Source: CAD feature listing. Evaluate the final solid. Frame: model axes, mm. A direction names the side the tool comes from. Give positions to 0.01 mm unless a question says otherwise; leave off trailing zeros. Write each loop counter-clockwise with the first axis right and the second up, starting at its lowest first coordinate (ties: lowest second). Pieces come first, ordered by that corner, then holes. Notation, with made-up numbers: M 5.25,-1 L 46.25,-1 A11 cw 46.25,5 Z; hole C 42,-11.5 d5. An arc over 180 degrees is marked long. Use CSV: the item, a comma, the result in double quotes. Start each with the question number.
from build123d import *

# Parameters (mm, degrees)
SKETCH1_R           = 19.75
BOSS_EXTRUDE1_DEPTH = 0.55


with BuildPart() as part:
    # Sketch1 → Boss-Extrude1 (new body)
    with BuildSketch(Plane(origin=(0, 0, 0), x_dir=(0, 0, -1), z_dir=(1, 0, 0))):
        Circle(SKETCH1_R)
        with BuildLine():
            Line((5.922649731, 1), (3.872983346, 1))
            ThreePointArc((3.872983346, 1), (0, 4), (-3.872983346, 1))
            Line((-3.872983346, 1), (-5.922649731, 1))
            Line((-5.922649731, 1), (-7.077350269, 1))
            Line((-7.077350269, 1), (-7.654700538, 0))
            Line((-7.654700538, 0), (-7.077350269, -1))
            Line((-7.077350269, -1), (-5.922649731, -1))
            Line((-5.922649731, -1), (-3.872983346, -1))
            ThreePointArc((-3.872983346, -1), (0, -4), (3.872983346, -1))
            Line((3.872983346, -1), (5.922649731, -1))
            Line((5.922649731, -1), (6.5, -1))
            Line((6.5, -1), (7.077350269, -1))
            Line((7.077350269, -1), (7.654700538, 0))
            Line((7.654700538, 0), (7.077350269, 1))
            Line((7.077350269, 1), (6.5, 1))
            Line((6.5, 1), (5.922649731, 1))
        make_face(mode=Mode.SUBTRACT)
    extrude(amount=BOSS_EXTRUDE1_DEPTH)


solid = part.part
1. Line query: probe 1 along Y at (x, z) = (0.1, 6); probe 2 along Y at (x, z) = (0.3, 1); probe 3 along Z at (x, y) = (0.35, 2.5). Output: solid intervals per line, ascending.
2. Section A-A on z = 0. Return loops of the section in (x, y).
3. Section D-D on y = 8.5. Return loops of the section in (x, z), then the cut area to 3 significant figures.
4. Section C-C on y = 3. Return loops of the section in (x, z), then the cut area to 3 significant figures.
5. Section B-B on x = 0.35. Return loops of the section in (y, z).
6. Access query for faces 1 (the flat face through (0.55, 5, 0)), 2 (the cylindrical face through (0.3, -4, 0.1)). Directions: +Z, -Z, +X, -X, +Y, -Y. A direction counts if a zero-diameter tool reaches every point of the face in a straight line with its end or side. Return the directions, or none.
7. Pull-direction query (Y, two-part tool) for faces 3 (the cylindrical face through (0.3, 4, -0.1)), 4 (the cylindrical face through (0.3, 13.3, 14.6)), 5 (the flat face through (0, 5, 0)); classes: released by +Y, released by -Y, zero draft, split by the parting line, or undercut.
Resolved:
1,probe 1,"y = -18.82 to -1, 1 to 18.82"
1,probe 2,"y = -19.72 to -3.87, 3.87 to 19.72"
1,probe 3,"z = -19.59 to -3.12, 3.12 to 19.59"
2,outline,"M 0,-19.75 L 0.55,-19.75 L 0.55,-4 L 0,-4 Z; M 0,4 L 0.55,4 L 0.55,19.75 L 0,19.75 Z"
3,outline,"M 0,-17.83 L 0.55,-17.83 L 0.55,17.83 L 0,17.83 Z"
3,area,"19.6 mm2"
4,outline,"M 0,-19.52 L 0.55,-19.52 L 0.55,-2.65 L 0,-2.65 Z; M 0,2.65 L 0.55,2.65 L 0.55,19.52 L 0,19.52 Z"
4,area,"18.6 mm2"
5,outline,"C 0,0 d39.5; hole M -1,-7.08 L 0,-7.65 L 1,-7.08 L 1,-3.87 A4 ccw 1,3.87 L 1,7.08 L 0,7.65 L -1,7.08 L -1,3.87 A4 ccw -1,-3.87 Z"
6,face 1,"+Z, -Z, +X, +Y, -Y"
6,face 2,"+X, -X"
7,face 3,"undercut"
7,face 4,"split by the parting line"
7,face 5,"zero draft"
